For this review, use the dimensioned drawing (mm, ordinates from the lowest corner) and the shaded views. Coordinates: 2 decimals unless noted, no trailing zeros. Write each loop counter-clockwise with the first axis right and the second up, starting at its lowest first coordinate (ties: lowest second). Pieces come first, ordered by that corner, then holes.
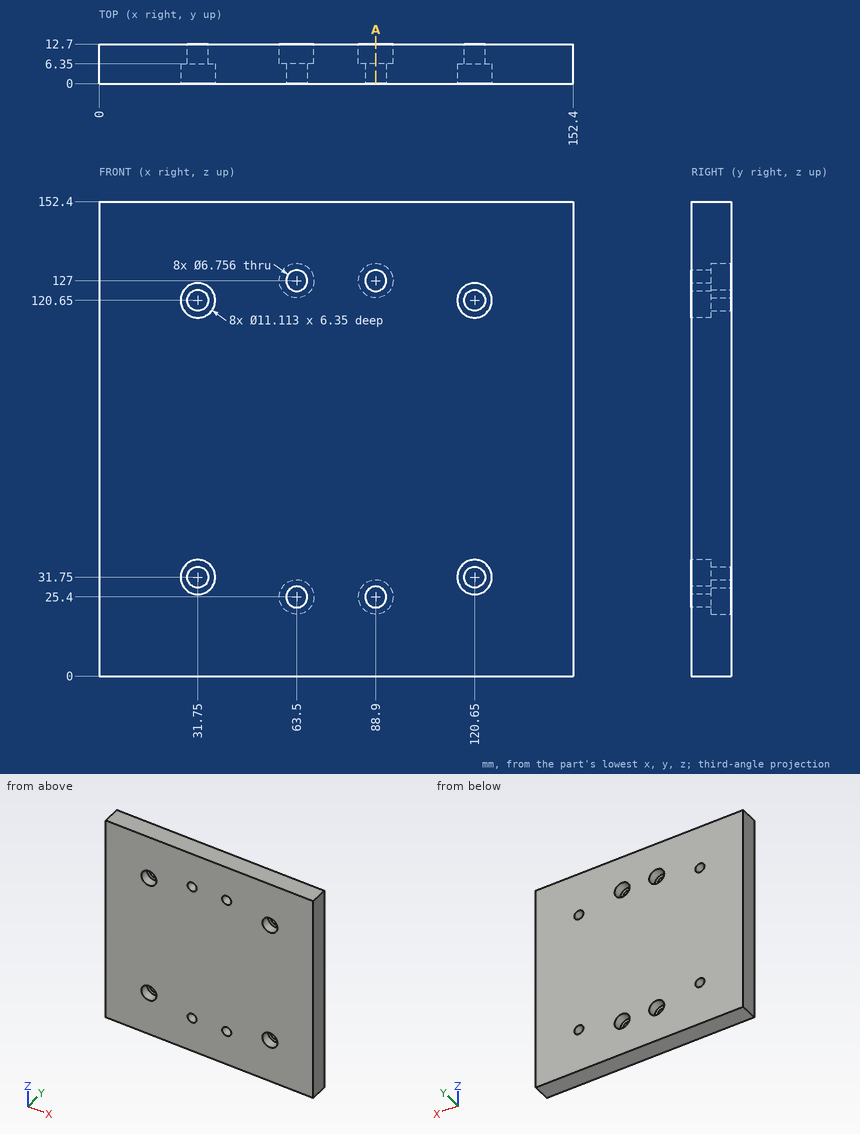
Item 1: Take a section at A-A, the plane x = 88.9. Write out the cut boundary in (y, z), plus the area to 3 significant figures.
Solved:
outline: (0, 0) - (12.7, 0) - (12.7, 19.84) - (6.35, 19.84) - (6.35, 22.02) - (0, 22.02) - close; (0, 28.78) - (6.35, 28.78) - (6.35, 30.96) - (12.7, 30.96) - (12.7, 121.44) - (6.35, 121.44) - (6.35, 123.62) - (0, 123.62) - close; (0, 130.38) - (6.35, 130.38) - (6.35, 132.56) - (12.7, 132.56) - (12.7, 152.4) - (0, 152.4) - close
area: 1,710 mm2
Item 2: For pin 1 (5.5 mm diameter, centred on x = 120.65, z = 120.65, fed in from +Y); pin 2 (3.5 mm diameter, centred on x = 122.5, z = 32, fed in from -Y); pin 3 (8 mm diameter, centred on x = 88.9, z = 127, fed in from +Y), all flat-tipped, find the tip position at first contact; note any pin that passes through.
Solved:
pin 1: passes through
pin 2: stops at y = 6.35
pin 3: stops at y = 6.35
Item 3: To check wall thickness, follow line 1 along X through (y, z) = (11, 31.75); line 2 along Z through (x, y) = (31.75, 3.5). State the ranges of each line that lie inside material, in increasing order.
Solved:
line 1: x = 0 to 28.37, 35.13 to 117.27, 124.03 to 152.4
line 2: z = 0 to 26.19, 37.31 to 115.09, 126.21 to 152.4
